```python
from build123d import *

# Parameters (mm, degrees)
SKETCH1_OUTSIDE_W  = 42.92
SKETCH1_OUTSIDE_H  = 42.92
CUT_EXTRUDE1_DEPTH = 17.51


with BuildPart() as part:
    # Sketch1 w/mock PCB → Revolve1 (revolve)
    with BuildSketch(Plane.XY, mode=Mode.PRIVATE) as revolve1_sk:
        with BuildLine():
            Line((0, 0), (-106.68, 0))
            Line((-106.68, 0), (-106.68, 7.14375))
            Line((-106.68, 7.14375), (-105.86085, 7.9629))
            Line((-105.86085, 7.9629), (-90.17, 7.9629))
            Line((-90.17, 7.9629), (-88.6714, 9.4615))
            Line((-88.6714, 9.4615), (-13.208, 9.4615))
            Line((-13.208, 9.4615), (-11.43, 7.6835))
            Line((-11.43, 7.6835), (-0.584426442, 7.6835))
            ThreePointArc((-0.584426442, 7.6835), (-0.146317327, 3.852847211), (0, 0))
        make_face()
    revolve(revolve1_sk.sketch.rotate(Axis((0, 0, 0), (1, 0, 0)), 90), axis=Axis((0, 0, 0), (1, 0, 0)))  # turned: the seam where the file's is

    # Sketch1 outside → Cut-Extrude1 (cut, through all)
    with BuildSketch(Plane(origin=(-90.17, 0, 0), x_dir=(0, 0, -1), z_dir=(1, 0, 0))):
        Rectangle(SKETCH1_OUTSIDE_W, SKETCH1_OUTSIDE_H)
        Polygon((4.124445986, 7.14375), (-4.124445986, 7.14375), (-8.248891971, 0), (-4.124445986, -7.14375), (4.124445986, -7.14375), (8.248891971, 0), align=None, mode=Mode.SUBTRACT)
    extrude(amount=-CUT_EXTRUDE1_DEPTH, mode=Mode.SUBTRACT)

    # Sketch2 → Cut-Revolve1 (revolve, cut)
    with BuildSketch(Plane.XY, mode=Mode.PRIVATE) as cut_revolve1_sk:
        Polygon((-98.464010462, 0), (-99.380554014, 1.5875), (-102.555554014, 1.5875), (-106.68, 3.96875), (-106.68, 0), align=None)
    revolve(cut_revolve1_sk.sketch.rotate(Axis((-106.68, 0, 0), (-1, 0, 0)), 270), axis=Axis((-106.68, 0, 0), (-1, 0, 0)), mode=Mode.SUBTRACT)  # turned: the seam where the file's is


solid = part.part
```
The model under review builds one solid part; all positions refer to its coordinate system, in mm. A direction names the side the tool comes from. Round coordinates to 2 decimals unless told otherwise and drop trailing zeros. Write each loop counter-clockwise with the first axis right and the second up, starting at its lowest first coordinate (ties: lowest second). Pieces come first, ordered by that corner, then holes.
(1) Mouldability with a two-part tool opening along Z and no side actions: class faces 4 (the cylindrical face through (-5.931, 6.817, 3.545)), 5 (the conical face through (-106.447, -6.361, 3.735)), 6 (the cylindrical face through (-100.99, -0.966, -1.26)), 7 (the conical face through (-98.623, -0.269, -0.06)) as +Z half, -Z half, draft (parallel to the pull), parting line (faces both ways), or undercut.
(2) Machinability: for faces 1 (the flat face through (-98.309, -3.615, -6.162)), 2 (the flat face through (-90.17, 3.6, 6.5)), 3 (the flat face through (-90.17, 3.8, -6.4)), which of the approach directions +Z, -Z, +X, -X, +Y, -Y give a long, thin tool a straight path to every point of the face, cutting with its end or side? Answer none if there is none.
(3) We need section B-B on x = -64.5. Give the boundary of the cut face in (y, z).
(4) We need section A-A on x = -95.5. Give the boundary of the cut face in (y, z).
(5) Insertion check: pin 1 (1.5 mm diameter, centred on x = -28.5, z = -4.5, fed in from +Y); pin 2 (2 mm diameter, centred on x = -49, z = 3, fed in from -Y); pin 3 (2 mm diameter, centred on x = -89, z = 6.5, fed in from +Y). Each pin has a flat end and moves straight along its axis. Give the tip position at first contact, or say it passes through.
(6) Wall thickness on L1, parallel to Y at x = -101.15, z = 0; L2, parallel to Y at x = -14, z = -0.5; L3, parallel to X at y = -0.5, z = 1: over which ranges is each line inside the solid? List them lowest first.
Findings below:
1. face 4: parting line
1. face 5: +Z half
1. face 6: undercut
1. face 7: undercut
2. face 1: -Z, -X, -Y
2. face 2: +Z, -X, +Y
2. face 3: -Z, -X, +Y
3. outline: circle Ø18.92 at (0, 0)
4. outline: (-7.14, -3.52) arc R7.96 ccw to (-6.62, -4.43) - (-0.53, -7.95) arc R7.96 ccw to (0.53, -7.95) - (6.62, -4.43) arc R7.96 ccw to (7.14, -3.52) - (7.14, 3.52) arc R7.96 ccw to (6.62, 4.43) - (0.53, 7.95) arc R7.96 ccw to (-0.53, 7.95) - (-6.62, 4.43) arc R7.96 ccw to (-7.14, 3.52) - close
5. pin 1: stops at y = 8.69
5. pin 2: stops at y = -9.25
5. pin 3: stops at y = 7.66
6. L1: y = -7.14 to -1.59, 1.59 to 7.14
6. L2: y = -9.45 to 9.45
6. L3: x = -99.11 to -0.01
